Design review of the part built by this model. Coordinates are the model's own, in mm. A direction names the side the tool comes from. Coordinates: 2 decimals unless noted, no trailing zeros. Write each loop counter-clockwise with the first axis right and the second up, starting at its lowest first coordinate (ties: lowest second). Pieces come first, ordered by that corner, then holes. Notation, with made-up numbers: (65, 55) - (101, 55) arc R18 ccw to (101, 89) - close; hole circle Ø10 at (-4.5, -16). An arc over 180 degrees is marked (long way). Answer as a JSON object with one key per item and string values.
```python
from build123d import *

# Parameters (mm, degrees)
SKETCH1_R           = 70
PLATE_DEPTH         = 12
SKETCH3_R           = 49.7
SKETCH3_R_2         = 43
SPIGOT_RING_DEPTH   = 10
CHAMFER_2_SIZE      = 0.8
SKETCH4_R           = 54.2
SKETCH4_R_2         = 50.8
FACE_GROOVE_DEPTH   = 2
FILLET1_R           = 0.2
ROD_HOLES_START     = -12
ROD_HOLES_OUTLINE_R = 2.75
ROD_HOLES_DEPTH     = 12
CHAMFER2_SIZE       = 0.8
P_C_D               = 10.2


# Read off the part's stored shape, not the designer's step: Rod_holes
with BuildPart() as part:
    # Sketch1 → PLATE (new body)
    with BuildSketch(Plane.XY):
        Circle(SKETCH1_R)
    extrude(amount=-PLATE_DEPTH)

    # Sketch3 → Spigot_Ring (add)
    with BuildSketch(Plane.XY):
        Circle(SKETCH3_R)
        Circle(SKETCH3_R_2, mode=Mode.SUBTRACT)
    extrude(amount=SPIGOT_RING_DEPTH)

    # Chamfer 2
    chamfer_2_edges = [part.edges().sort_by_distance(p)[0] for p in [
        (-49.7, 0, 10),
    ]]
    chamfer(chamfer_2_edges, length=CHAMFER_2_SIZE)

    # Sketch4 → Face_Groove (cut)
    with BuildSketch(Plane.XY):
        Circle(SKETCH4_R)
        Circle(SKETCH4_R_2, mode=Mode.SUBTRACT)
    extrude(amount=-FACE_GROOVE_DEPTH, mode=Mode.SUBTRACT)

    # Fillet1
    fillet1_edges = [part.edges().sort_by_distance(p)[0] for p in [
        (-54.2, 0, -2),
        (-50.8, 0, -2),
    ]]
    fillet(fillet1_edges, radius=FILLET1_R)

    # Rod_holes outline → Rod_holes (cut)
    with BuildSketch(Plane.XY.offset(ROD_HOLES_START)):
        with Locations((-62, 0)):
            Circle(ROD_HOLES_OUTLINE_R)
        with Locations((0, -62)):
            Circle(ROD_HOLES_OUTLINE_R)
        with Locations((62, 0)):
            Circle(ROD_HOLES_OUTLINE_R)
        with Locations((0, 62)):
            Circle(ROD_HOLES_OUTLINE_R)
    extrude(amount=ROD_HOLES_DEPTH, mode=Mode.SUBTRACT)

    # Chamfer2
    chamfer2_edges = [part.edges().sort_by_distance(p)[0] for p in [
        (-70, 0, 0),
        (-64.75, 0, 0),
        (-64.75, 0, -12),
        (-2.75, -62, 0),
        (-2.75, -62, -12),
        (59.25, 0, 0),
        (59.25, 0, -12),
        (-70, 0, -12),
        (-2.75, 62, 0),
        (-2.75, 62, -12),
    ]]
    chamfer(chamfer2_edges, length=CHAMFER2_SIZE)

    # P_C (through all)
    with Locations(Plane(origin=(0, 0, -12), x_dir=(-1, 0, 0), z_dir=(0, 0, -1))):
        with Locations((0, 0)):
            Hole(P_C_D / 2)


solid = part.part
```
(1) For pin 1 (8 mm diameter, centred on y = -2, z = -5, fed in from +X); pin 2 (6.5 mm diameter, centred on x = -62, y = 0, fed in from +Z); pin 3 (10 mm diameter, centred on x = 35.5, z = -1.5, fed in from +Y); pin 4 (6.5 mm diameter, centred on x = 62, y = 0, fed in from -Z), all flat-tipped, find the tip position at first contact; note any pin that passes through.
Solved:
{"pin 1": "stops at x = 70", "pin 2": "stops at z = -0.3", "pin 3": "stops at y = 63.01", "pin 4": "stops at z = -11.7"}
(2) Take a section at A-A, the plane z = -5. Write out the cut boundary in (x, y), and give its area (3 significant figures).
Solved:
{"outline": "circle Ø140 at (0, 0); hole circle Ø5.5 at (-62, 0); hole circle Ø10.2 at (0, 0); hole circle Ø5.5 at (0, -62); hole circle Ø5.5 at (0, 62); hole circle Ø5.5 at (62, 0)", "area": "15,200 mm^2"}
(3) The part is to be moulded in two halves that separate along Y. For faces 1 (the face through (-39.44, -30.24, 4.54)), 2 (the face through (9, 1, 0)), 3 (the face through (-1, -14, -12)), say which applies: pulls with the +Y half, pulls with the -Y half, needs draft (parallel to the pull), parting line crosses it, or undercut.
Solved:
{"face 1": "parting line crosses it", "face 2": "undercut", "face 3": "needs draft"}
(4) To check wall thickness, follow line 1 (Y direction, x = 0, z = -5.75); line 2 (Y direction, x = 0, z = 7.25); line 3 (X direction, y = 16.5, z = -0.75). State the ranges of each line that lie inside material, in increasing order. Write a range as from..to.
Solved:
{"line 1": "y = -70..-64.75, -59.25..-5.1, 5.1..59.25, 64.75..70", "line 2": "y = -49.7..-43, 43..49.7", "line 3": "x = -67.98..-51.63, -48.05..48.05, 51.63..67.98"}
(5) Tool access review of faces 4 (the face through (-0.358, -59.273, -6.073)), 5 (the face through (-5.598, 42.634, 4.93)): name each direction out of +Z, -Z, +X, -X, +Y, -Y from which nothing blocks a thin tool from reaching the whole face with its end or side.
Solved:
{"face 4": "+Z, -Z", "face 5": "+Z"}
(6) Take a section at B-B, the plane x = 0. Give the number of separate pieces and of enclosed holes in the cut face, and give its area (3 significant figures).
Solved:
{"separate pieces": "4", "enclosed holes": "0", "area": "1,540 mm^2"}
(7) Take a section at D-D, the plane z = 6.75. Write out the cut boundary in (x, y).
Solved:
{"outline": "circle Ø99.4 at (0, 0); hole circle Ø86 at (0, 0)"}
